Read the model definition and answer for the solid it produces. Units are mm, in the model's axes. A direction names the side the tool comes from. Coordinates: 2 decimals unless noted, no trailing zeros. Loops run counter-clockwise (first coordinate to the right, second up) from the corner with the lowest first, then second, coordinate; pieces in that order, holes last. Notation, with made-up numbers: (25, 39) -> (70, 39) arc R31 ccw to (70, 78) -> close; hole circle Ø1 at (10.25, 79.25). An arc over 180 degrees is marked (long way). Answer as a JSON object with one key per item and string values. Group by question number.
1) Which of the six approach directions +Z, -Z, +X, -X, +Y, -Y give full straight-line access (tool end or side, diameter ignored) to faces 4 (the face through (-15.62, 2.46, 3.47)), 5 (the face through (-18, 1, -0.75)), 6 (the face through (0.1, 0, -16.5)), 7 (the face through (9.76, 31.31, 2.17))?
2) Section B-B, the plane x = 2 is taken. Give the vertices of the cut face in (y, z).
3) Section D-D, the plane x = -8.5 is taken. Give the vertices of the cut face in (y, z).
4) Determine the mould class of faces 1 (the face through (-5.902, 22.185, -18.743)), 2 (the face through (-5, 45, 9)), 3 (the face through (0, 18, -2)) for opening direction Z: released by +Z, released by -Z, zero draft, split by the parting line, or undercut.
5) Section A-A, the plane y = 12.5 is taken. Give the vertices of the cut face in (x, z), plus the area to 3 significant figures.
6) Consider probe 1 along Z at (x, y) = (0.5, 25); probe 2 along X at (y, z) = (3.4, 0); probe 3 along X at (y, z) = (15.25, 0). Determine where each line is inside the solid, lowest interval first. Write a range as [from, to].
7) Flat-ended cylindrical pins translate along their axes: P1, Ø6, axis at x = -15.5, y = 8, coming from the -Z side; P2, Ø8, axis at x = 6, y = 20.5, coming from the -Z side; P3, Ø1.7, axis at x = 17, z = 0, coming from the -Y side; P4, Ø8, axis at y = 6.5, z = 15.5, coming from the +X side. Find the tip coordinate at first contact, or state that the pin passes through.
8) Section C-C, the plane y = 25.5 is taken. Give the vertices of the cut face in (x, z).
from build123d import *

# Parameters (mm, degrees)
SKETCH_1_R          = 19.65
SKETCH_1_R_2        = 10
EXTRUDE_1_DEPTH     = 45
SKETCH_2_R          = 10
SKETCH_2_R_2        = 0.5
EXTRUDE_2_DEPTH     = 18
SKETCH_3_R          = 16
CUT_EXTRUDE_1_DEPTH = 5
SKETCH_5_W          = 1.5
SKETCH_5_H          = 1.5
CUT_EXTRUDE_2_DEPTH = 63.5


with BuildPart() as part:
    # Sketch 1 → Extrude 1 (new body)
    with BuildSketch(Plane(origin=(0, 0, 0), x_dir=(1, 0, 0), z_dir=(0, 1, 0))):
        with Locations(Location((0, 0, 0), (0, 0, 90))):
            Circle(SKETCH_1_R)
        with Locations(Location((0, 0, 0), (0, 0, 90))):
            Circle(SKETCH_1_R_2, mode=Mode.SUBTRACT)
    extrude(amount=EXTRUDE_1_DEPTH)

    # Sketch 2 → Extrude 2 (add)
    with BuildSketch(Plane.XZ):
        with Locations(Location((0, 0, 0), (0, 0, 270))):
            Circle(SKETCH_2_R)
        with Locations(Location((0, 0, 0), (0, 0, 270))):
            Circle(SKETCH_2_R_2, mode=Mode.SUBTRACT)
    extrude(amount=-EXTRUDE_2_DEPTH)

    # Sketch 3 → Cut-Extrude 1 (cut)
    with BuildSketch(Plane.XZ):
        with Locations(Location((0, 0, 0), (0, 0, 270))):
            Circle(SKETCH_3_R)
    extrude(amount=-CUT_EXTRUDE_1_DEPTH, mode=Mode.SUBTRACT)

    # Sketch 5 → Cut-Extrude 2 (cut, symmetric)
    with BuildSketch(Plane(origin=(0, 45, 0), x_dir=(0, 0, 1), z_dir=(-1, 0, 0))):
        with Locations((0, -44.25)):
            Rectangle(SKETCH_5_W, SKETCH_5_H)
    extrude(amount=CUT_EXTRUDE_2_DEPTH, both=True, mode=Mode.SUBTRACT)


solid = part.part
Determined:
{
 "1": {"face 4": "-Y", "face 5": "+X, -X, -Y", "face 6": "+Z, -Z, +X, -X, -Y", "face 7": "+Y"},
 "2": {"outline": "(0, -19.55) -> (45, -19.55) -> (45, -9.8) -> (18, -9.8) -> (18, 9.8) -> (45, 9.8) -> (45, 19.55) -> (0, 19.55) -> (0, 15.87) -> (5, 15.87) -> (5, -15.87) -> (0, -15.87) -> close"},
 "3": {"outline": "(0, -17.72) -> (45, -17.72) -> (45, -5.27) -> (18, -5.27) -> (18, 5.27) -> (45, 5.27) -> (45, 17.72) -> (0, 17.72) -> (0, 13.56) -> (5, 13.56) -> (5, -13.56) -> (0, -13.56) -> close"},
 "4": {"face 1": "split by the parting line", "face 2": "zero draft", "face 3": "undercut"},
 "5": {"outline": "circle Ø39.3 at (0, 0); hole circle Ø1 at (0, 0)", "area": "1,210 mm²"},
 "6": {"probe 1": "[-19.64, -9.99], [9.99, 19.64]", "probe 2": "[-19.65, -16], [16, 19.65]", "probe 3": "[-19.65, -0.5], [0.5, 19.65]"},
 "7": {"P1": "z = -15.16", "P2": "z = -19.55", "P3": "y = 0", "P4": "x = 15.93"},
 "8": {"outline": "circle Ø39.3 at (0, 0); hole circle Ø20 at (0, 0)"}
}
